Check sheet for the modelled part. Datum: model origin and axes. Units: mm. Round coordinates to 2 decimals unless told otherwise and drop trailing zeros. Write each loop counter-clockwise with the first axis right and the second up, starting at its lowest first coordinate (ties: lowest second). Pieces come first, ordered by that corner, then holes. Notation, with made-up numbers: M 54,14 L 98,14 A7 ccw 98,24 Z; hole C 89.25,46.5 d4. An arc over 180 degrees is marked long. Answer in a Markdown table with one row per item.
Autodesk Inventor part; units mm, degrees
ref_plane "Work Plane1" through (139.7, 101.6, 0) normal (1, 0, 0) x (0, 0, -1)
ref_plane "Work Plane2" through (0, 0, 50.8) normal (0, 0, 1) x (1, 0, 0)
ref_plane "YZ Plane" through (0, 0, 0) normal (1, 0, 0) x (0, 1, 0)
sketch "Sketch1" plane through (0, 0, 0) normal (0, 0, 1) x (1, 0, 0)
  line L0 (0, 0) -> (279.4, 0)
  line L1 (279.4, 0) -> (279.4, 279.4)
  line L2 (279.4, 279.4) -> (0, 279.4)
  line L3 (0, 279.4) -> (0, 0)
  circle A0 centre (139.7, 134.62) radius 30.1752
  circle A1 centre (139.7, 228.6) radius 30.1752
  circle A2 centre (66.2235, 193.2156) radius 30.1752
  circle A3 centre (48.0763, 113.7075) radius 30.1752
  circle A4 centre (98.9236, 49.9469) radius 30.1752
  circle A5 centre (180.4764, 49.9469) radius 30.1752
  circle A6 centre (231.3237, 113.7075) radius 30.1752
  circle A7 centre (213.1765, 193.2156) radius 30.1752
  dimension "d0" = 279.4
  dimension "d1" = 279.4
  dimension "d2" = 60.3504
  dimension "d3" = 60.3504
  dimension "d22" = 360
extrude "Extrusion1" add sketch "Sketch1" along normal blind 101.6
fillet "Fillet1" radius 101.6 4 edges at (279.4, 279.4, 50.8) (0, 279.4, 50.8) (279.4, 0, 50.8) (0, 0, 50.8)
ref_plane "Work Plane1" through (139.7, 101.6, 0) normal (1, 0, 0) x (0, 0, -1)
ref_plane "Work Plane2" through (0, 0, 50.8) normal (0, 0, 1) x (1, 0, 0)
sketch "Sketch2" plane through (279.4, 101.6, 0) normal (1, 0, 0) x (0, 0, -1)
  line L0 (0, 0) -> (-101.6, 0)
  line L1 (0, 0) -> (0, 76.2)
  line L2 (-101.6, 76.2) -> (0, 76.2)
  line L3 (-101.6, 0) -> (-101.6, 76.2)
  circle A0 centre (-50.8, 38.1) radius 12.7
  point P0 (0, -101.6)
  dimension "d14" = 25.4
sketch "Sketch3" plane through (0, 101.6, 0) normal (-1, 0, 0) x (0, 0, 1)
  line L0 (101.6, 0) -> (0, 0)
  line L1 (101.6, 76.2) -> (101.6, 0)
  line L2 (0, 76.2) -> (101.6, 76.2)
  line L3 (0, 76.2) -> (0, 0)
  circle A0 centre (50.8, 38.1) radius 12.7
  point P0 (0, -101.6)
  dimension "d15" = 25.4
properties part number "ShooterMount-1in"
1. Section check A-A, the plane x = 139.7. Record the cut outline in (y, z).
Found:
| item | result |
|---|---|
| outline | M 0,0 L 104.44,0 L 104.44,101.6 L 0,101.6 Z; M 164.8,0 L 198.42,0 L 198.42,101.6 L 164.8,101.6 Z; M 258.78,0 L 279.4,0 L 279.4,101.6 L 258.78,101.6 Z |
2. Draft check along Y on faces 1 (the face through (259.2, 125.26, 50.09)), 2 (the face through (209.258, 40.883, 50.089)), 3 (the face through (169, 111, 0)), 4 (the face through (250.428, 248.848, 51.511)). Enter one of: +Y half, -Y half, draft (parallel to the pull), parting line (faces both ways), or undercut.
Found:
| item | result |
|---|---|
| face 1 | undercut |
| face 2 | undercut |
| face 3 | draft |
| face 4 | +Y half |
3. Section check D-D, the plane z = 62. Count the separate pieces of the cut face and the enclosed holes in it, and give its area (3 significant figures).
Found:
| item | result |
|---|---|
| separate pieces | 1 |
| enclosed holes | 8 |
| area | 46,300 mm2 |
4. Section check C-C, the plane y = 236.5. Record the cut outline in (x, z), and give its area (3 significant figures).
Found:
| item | result |
|---|---|
| outline | M 18.67,0 L 110.58,0 L 110.58,101.6 L 18.67,101.6 Z; M 168.82,0 L 260.73,0 L 260.73,101.6 L 168.82,101.6 Z |
| area | 18,700 mm2 |
5. Scan lines: L1, parallel to Y at x = 139, z = 24; L2, parallel to Y at x = 139.7, z = 78.5; L3, parallel to X at y = 219.5, z = 54. Record each from-to range of solid material in increasing order.
Found:
| item | result |
|---|---|
| L1 | y = 0 to 104.45, 164.79 to 198.43, 258.77 to 279.4 |
| L2 | y = 0 to 104.44, 164.8 to 198.42, 258.78 to 279.4 |
| L3 | x = 8.95 to 51.4, 81.04 to 110.93, 168.47 to 198.36, 228 to 270.45 |
6. Section check B-B, the plane y = 134.62. Record the cut outline in (x, z).
Found:
| item | result |
|---|---|
| outline | M 0,0 L 26.32,0 L 26.32,101.6 L 0,101.6 Z; M 69.83,0 L 109.52,0 L 109.52,101.6 L 69.83,101.6 Z; M 169.88,0 L 209.57,0 L 209.57,101.6 L 169.88,101.6 Z; M 253.08,0 L 279.4,0 L 279.4,101.6 L 253.08,101.6 Z |
7. Go/stop test with flat-tipped pins: pin 1 (1.5 mm diameter, centred on x = 227.5, z = 51.5, fed in from -Y); pin 2 (12 mm diameter, centred on x = 205, z = 15.5, fed in from +Y); pin 3 (6 mm diameter, centred on y = 145, z = 13.5, fed in from -X); pin 4 (2 mm diameter, centred on y = 30, z = 85.5, fed in from +X). Record where each tip stops, or that it passes through.
Found:
| item | result |
|---|---|
| pin 1 | stops at y = 12.57 |
| pin 2 | stops at y = 277.16 |
| pin 3 | stops at x = 0 |
| pin 4 | stops at x = 250.86 |
